Autodesk Inventor part; units mm, degrees
ref_plane "YZ Plane" through (0, 0, 0) normal (1, 0, 0) x (0, 1, 0)
ref_plane "XZ Plane" through (0, 0, 0) normal (0, 1, 0) x (-1, 0, 0)
ref_plane "XY Plane" through (0, 0, 0) normal (0, 0, 1) x (1, 0, 0)
sketch "Sketch1" plane through (0, 0, 0) normal (0, 0, 1) x (1, 0, 0)
  line L0 (0, 0) -> (0, 85.852)
  line L1 (0, 85.852) -> (2.54, 85.852)
  line L2 (2.54, 85.852) -> (2.54, 83.312)
  line L3 (5.5626, 79.0463) -> (5.5626, 0)
  line L4 (5.5626, 0) -> (0, 0)
  line L5 (2.54, 83.312) -> (4.4196, 83.312)
  line L6 (4.4196, 83.312) -> (5.5626, 79.0463)
  dimension "d0" = 83.312
  dimension "d1" = 2.54
  dimension "d2" = 75
  dimension "d3" = 1.143
  dimension "d4" = 5.5626
  dimension "d5" = 2.54
revolve "Revolution1" add sketch "Sketch1" angle 360 about axis through (0, 0, 0) along (0, 1, 0)
hole "Hole1" at (0, 0, 0) direction (0, 1, 0) diameter 2.6416 depth 15.0876 tip angle 118
hole "Hole2" at (0, 85.852, 0) direction (0, -1, 0) diameter 2.6416 depth 15.0876 tip angle 118
properties part number "kinect standoff" material "Aluminum-6061"
Build history of the part. All positions in model axes, mm. A direction names the side the tool comes from. Give positions to 0.01 mm unless a question says otherwise; leave off trailing zeros. Order: outer loops, then holes, each group sorted by start corner. A loop starts at its lowest first (then second) coordinate and runs counter-clockwise, first axis right, second up. Notation, with made-up numbers: M 66,45.5 L 116,45.5 A7 ccw 116,55.5 Z; hole C 85,34 d4. An arc over 180 degrees is marked long. Return JSON: item names as keys, results as strings.
Q1. Two-plate mould, pull along X, no slides. Class faces 3 (the face through (-4.614, 82.571, 0.203)), 4 (the face through (2, 83.312, 2)), 5 (the face through (0.8, 7.65, 1.05)): pulls with the +X half, pulls with the -X half, needs draft (parallel to the pull), parting line crosses it, or undercut.
Answer list:
{"face 3": "parting line crosses it", "face 4": "needs draft", "face 5": "undercut"}
Q2. Wall check: probe 1 along X at (y, z) = (8, 0); probe 2 along Y at (x, z) = (3.25, 0.25). Give the ranges that are in metal, low to high. Write a range as from..to.
Answer list:
{"probe 1": "x = -5.56..-1.32, 1.32..5.56", "probe 2": "y = 0..83.31"}
Q3. Band-saw the part on A-A (y = 34). Give the cut face in (x, z), then the cut area to 3 significant figures.
Answer list:
{"outline": "C 0,0 d11.13", "area": "97.2 mm^2"}
Q4. 3-axis set-ups, long thin cutter, end or side, ignore diameter. For faces 1 (the face through (1.1, 85.852, 1.1)), 2 (the face through (-0.33, 84.56, 2.52)): which of +Z, -Z, +X, -X, +Y, -Y reach the whole face in a straight line?
Answer list:
{"face 1": "+Z, -Z, +X, -X, +Y", "face 2": "+Y"}
Q5. Flat gauge pins, fed straight in: pin 1 (3 mm diameter, centred on y = 76.5, z = -3.5, fed in from +X); pin 2 (2.5 mm diameter, centred on x = 0, z = 0, fed in from -Y); pin 3 (5 mm diameter, centred on x = 3, y = 76, fed in from +Z). Where does each tip first touch, or does it go through?
Answer list:
{"pin 1": "stops at x = 5.19", "pin 2": "stops at y = 15.13", "pin 3": "stops at z = 5.54"}
